Autodesk Inventor part; units mm, degrees
ref_plane "YZ Plane" through (0, 0, 0) normal (1, 0, 0) x (0, 1, 0)
ref_plane "XZ Plane" through (0, 0, 0) normal (0, 1, 0) x (-1, 0, 0)
ref_plane "XY Plane" through (0, 0, 0) normal (0, 0, 1) x (1, 0, 0)
sketch "Sketch1" plane through (0, 0, 0) normal (0, 1, 0) x (-1, 0, 0)
  line L0 (0, 0) -> (0, 7.5)
  line L1 (0, 7.5) -> (7.5, 7.5)
  line L2 (7.5, 7.5) -> (7.5, -7.5)
  line L3 (7.5, -7.5) -> (-7.5, -7.5)
  line L4 (-7.5, -7.5) -> (-7.5, 7.5)
  line L5 (-7.5, 7.5) -> (0, 7.5)
  dimension "d0" = 7.5
  dimension "d1" = 7.5
  dimension "d2" = 15
  dimension "d3" = 15
extrude "Extrusion1" add sketch "Sketch1" along normal blind 3
fillet "Fillet1" radius 2 4 edges at (7.5, 1.5, 7.5) (7.5, 1.5, -7.5) (-7.5, 1.5, 7.5) (-7.5, 1.5, -7.5)
sketch "Sketch2" plane through (0, 3, 0) normal (0, 1, 0) x (1, 0, 0)
  circle A0 centre (0, 0) radius 2
  dimension "d7" = 4
extrude "Extrusion2" cut sketch "Sketch2" against normal blind 3
sketch "Sketch3" plane through (0, 3, 0) normal (0, 1, 0) x (1, 0, 0)
  line L0 (0, 0) -> (7.5, 0)
  line L1 (7.5, -5.5) -> (7.5, 5.5)
  line L2 (7.5, 0) -> (4.5, 0)
  line L3 (4.5, 0) -> (4.5, 4.5)
  line L4 (4.5, 4.5) -> (4.5, -4.5)
  line L5 (4.5, -4.5) -> (-4.5, -4.5)
  line L6 (-4.5, -4.5) -> (-7.5, -4.5)
  line L7 (-7.5, 5.5) -> (-7.5, -5.5)
  line L8 (4.5, 4.5) -> (4.5, 7.5)
  line L9 (5.5, 7.5) -> (-5.5, 7.5)
  line L10 (4.5, 7.5) -> (5.5, 7.5)
  line L11 (7.5, 5.5) -> (7.5, -5.5)
  line L12 (-5.5, -7.5) -> (5.5, -7.5)
  line L13 (5.5, -7.5) -> (-5.5, -7.5)
  arc A0 (7.5, 5.5) -> (5.5, 7.5) centre (5.5, 5.5) ccw
  arc A1 (7.5, 5.5) -> (5.5, 7.5) centre (5.5, 5.5) ccw
  arc A2 (5.5, -7.5) -> (7.5, -5.5) centre (5.5, -5.5) ccw
  arc A3 (5.5, -7.5) -> (7.5, -5.5) centre (5.5, -5.5) ccw
  line L14 (-7.5, -4.5) -> (-7.5, -5.5)
  arc A4 (-7.5, -5.5) -> (-5.5, -7.5) centre (-5.5, -5.5) ccw
  arc A5 (-7.5, -5.5) -> (-5.5, -7.5) centre (-5.5, -5.5) ccw
  dimension "d10" = 3
  dimension "d11" = 4.5
  dimension "d12" = 9
  dimension "d13" = 9
  dimension "d14" = 3
extrude "Extrusion3" add sketch "Sketch3" along normal blind 10
properties part number "legs"
Geometry check sheet. Reference: the model listing, model coordinates, mm. A direction names the side the tool comes from. Give positions to 0.01 mm unless a question says otherwise; leave off trailing zeros. Loops run counter-clockwise (first coordinate to the right, second up) from the corner with the lowest first, then second, coordinate; pieces in that order, holes last. Notation, with made-up numbers: (15, 3.25) -> (70, 3.25) arc R14 cw to (70, 29.25) -> close; hole circle Ø8 at (-17, 34.25). An arc over 180 degrees is marked (long way). Answer in a Markdown table with one row per item. Add a question column.
1) Cross-section at C-C on y = 1. Record the boundary of the cut face in (x, z).
2) Cross-section at D-D on y = 3.75. Record the boundary of the cut face in (x, z).
3) Gauge pin test, flat end, axial feed: P1, Ø5, axis at x = -1.5, z = -4, coming from the +Y side. Record the tip position at first contact, or that the pin passes through.
4) Material ranges on probe 1 along Z at (x, y) = (0, 2.1); probe 2 along X at (y, z) = (10.75, 0.75), recorded low to high. Write a range as from..to.
5) Cross-section at B-B on z = 0. Record the boundary of the cut face in (x, y), and give its area (3 significant figures).
6) Set-up check for faces 1 (the face through (4.5, 8, -1)), 2 (the face through (0, 6, 7.5)): record each of +Z, -Z, +X, -X, +Y, -Y from which the full face is reachable in a straight line by a thin tool's end or side.
7) Cross-section at A-A on x = 0. Record the boundary of the cut face in (y, z), and give its area (3 significant figures).
8) Draft check along Z on faces 3 (the face through (-1, 8, 4.5)), 4 (the face through (-7.5, 2.6, 1.2)), 5 (the face through (0, 2, 2)). Enter one of: pulls with the +Z half, pulls with the -Z half, needs draft (parallel to the pull), parting line crosses it, or undercut.
Outcome:
| question | item | result |
|---|---|---|
| 1 | outline | (-7.5, -5.5) arc R2 ccw to (-5.5, -7.5) -> (5.5, -7.5) arc R2 ccw to (7.5, -5.5) -> (7.5, 5.5) arc R2 ccw to (5.5, 7.5) -> (-5.5, 7.5) arc R2 ccw to (-7.5, 5.5) -> close; hole circle Ø4 at (0, 0) |
| 2 | outline | (-7.5, 4.5) -> (4.5, 4.5) -> (4.5, -7.5) -> (5.5, -7.5) arc R2 ccw to (7.5, -5.5) -> (7.5, 5.5) arc R2 ccw to (5.5, 7.5) -> (-5.5, 7.5) arc R2 ccw to (-7.5, 5.5) -> close |
| 3 | P1 | stops at y = 3 |
| 4 | probe 1 | z = -7.5..-2, 2..7.5 |
| 4 | probe 2 | x = 4.5..7.5 |
| 5 | outline | (-7.5, 0) -> (-2, 0) -> (-2, 3) -> (-7.5, 3) -> close; (2, 0) -> (7.5, 0) -> (7.5, 13) -> (4.5, 13) -> (4.5, 3) -> (2, 3) -> close |
| 5 | area | 63.0 mm^2 |
| 6 | face 1 | -Z, -X, +Y |
| 6 | face 2 | +Z, +X, -X, +Y, -Y |
| 7 | outline | (0, -7.5) -> (3, -7.5) -> (3, -2) -> (0, -2) -> close; (0, 2) -> (3, 2) -> (3, 4.5) -> (13, 4.5) -> (13, 7.5) -> (0, 7.5) -> close |
| 7 | area | 63.0 mm^2 |
| 8 | face 3 | pulls with the -Z half |
| 8 | face 4 | needs draft |
| 8 | face 5 | undercut |
